Here's how the part is built. I have some questions about the finished solid (model axes, mm). Face numbers are marked on the shaded views. A direction names the side the tool comes from. Coordinates: 2 decimals unless noted, no trailing zeros. Order: outer loops, then holes, each group sorted by start corner. A loop starts at its lowest first (then second) coordinate and runs counter-clockwise, first axis right, second up. Notation, with made-up numbers: (34.5, -20.75) - (70.5, -20.75) arc R14 ccw to (70.5, -11.75) - close; hole circle Ø2 at (53.25, 82). An arc over 180 degrees is marked (long way). Use CSV: the item, a comma, the result in double quotes. Start each with the question number.
from build123d import *

# Parameters (mm, degrees)
F0_W      = 39.88
F0_H      = 19.82
F1_DEPTH  = 26.67
F2_W      = 6.48
F2_H      = 19.82
F2_W_2    = 39.88
F3_DEPTH  = 2
F4_W      = 39.88
F4_H      = 19.82
F5_DEPTH  = 7.35
F6_R      = 6
F7_DEPTH  = 1.8
F8_R      = 3
F8_R_2    = 1.3258580477
F9_DEPTH  = 4.05
F10_R     = 2.19
F11_DEPTH = 25
F12_R     = 2


with BuildPart() as f1:
    # F0 (on Top) → F1 (new body)
    with BuildSketch(Plane.XY):
        with Locations((19.94, 9.91)):
            Rectangle(F0_W, F0_H)
    extrude(amount=F1_DEPTH)

    # F2 (on face) → F3 (join)
    with BuildSketch(Plane.XY.offset(26.67)):
        with Locations((-3.24, 9.91)):
            Rectangle(F2_W, F2_H)
        with Locations((19.94, 9.91)):
            Rectangle(F2_W_2, F2_H)
        with Locations((43.12, 9.91)):
            Rectangle(F2_W, F2_H)
    extrude(amount=F3_DEPTH)

    # F4 (on face) → F5 (join)
    with BuildSketch(Plane.XY.offset(28.67)):
        with Locations((19.94, 9.91)):
            Rectangle(F4_W, F4_H)
    extrude(amount=F5_DEPTH)

    # F6 (on face) → F7 (join)
    with BuildSketch(Plane.XY.offset(36.02)):
        with Locations((9.66, 9.91)):
            Circle(F6_R)
    extrude(amount=F7_DEPTH)

    # F8 (on face) → F9 (join)
    with BuildSketch(Plane.XY.offset(37.82)):
        with Locations((9.66, 9.91)):
            Circle(F8_R)
        with Locations((9.66, 9.91)):
            Circle(F8_R_2, mode=Mode.SUBTRACT)
    extrude(amount=F9_DEPTH)

    # F10 (on face) → F11 (cut)
    with BuildSketch(Plane.XY.offset(28.67)):
        with Locations((-3.81, 4.825)):
            Circle(F10_R)
        with Locations((-3.81, 14.995)):
            Circle(F10_R)
        with Locations((43.69, 4.825)):
            Circle(F10_R)
        with Locations((43.69, 14.995)):
            Circle(F10_R)
    extrude(amount=-F11_DEPTH, mode=Mode.SUBTRACT)

    # F12
    f12_edges = [f1.edges().sort_by_distance(p)[0] for p in [
        (-6.48, 19.82, 27.67),
        (46.36, 19.82, 27.67),
        (46.36, 0, 27.67),
        (-6.48, 0, 27.67),
    ]]
    fillet(f12_edges, radius=F12_R)


solid = f1.part
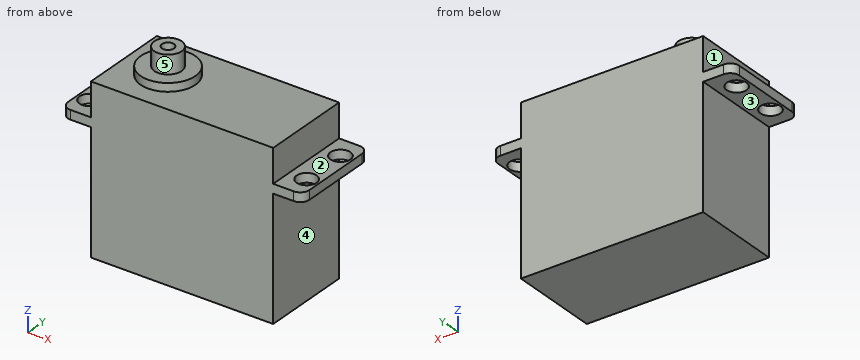
Item 1: For pin 1 Ø5 at (x, y) = (43.69, 14.995) entering from +Z; pin 2 Ø2 at (y, z) = (14, 33) entering from -X; pin 3 Ø10 at (x, y) = (18.5, 12) entering from +Z; pin 4 Ø2.5 at (x, y) = (-3.81, 4.825) entering from -Z, each with a flat end and sliding along its axis, tell me the tip position at first contact or that it passes through.
Item 2: Please list where these lines run through material, in increasing order: line 1 along Y through (x, z) = (43.69, 27.8) (3 decimals); line 2 along Y through (x, z) = (-3, 27); line 3 along X through (y, z) = (2.75, 9). Write a range as from..to.
Item 3: Suppose I cut it at D-D on x = 9.66. Write out the boundary of the cut face in (y, z), then the cut area to 3 significant figures.
Item 4: Suppose I cut it at A-A on x = -3.81. Write out the boundary of the cut face in (y, z) (3 decimals).
Item 5: Suppose I cut it at C-C on z = 28. Write out the boundary of the cut face in (x, y) (3 decimals).
Item 6: Suppose I cut it at B-B on y = 9.91. Write out the boundary of the cut face in (x, z).
Item 7: For the marked faces 1, 2, 3, 4 and 5, which set-ups out of +Z, -Z, +X, -X, +Y, -Y let a thin tool reach every point of the face, with its end or its side?
Here are the results:
1,pin 1,"z = 28.67"
1,pin 2,"x = 0"
1,pin 3,"z = 37.82"
1,pin 4,"through"
2,line 1,"0..2.635, 7.015..12.805, 17.185..19.82"
2,line 2,"0..2.79, 6.86..12.96, 17.03..19.82"
2,line 3,"0..39.88"
3,outline,"(0, 0) - (19.82, 0) - (19.82, 36.02) - (15.91, 36.02) - (15.91, 37.82) - (12.91, 37.82) - (12.91, 41.87) - (11.24, 41.87) - (11.24, 37.82) - (8.58, 37.82) - (8.58, 41.87) - (6.91, 41.87) - (6.91, 37.82) - (3.91, 37.82) - (3.91, 36.02) - (0, 36.02) - close"
3,area,"749 mm^2"
4,outline,"(0, 26.67) - (2.635, 26.67) - (2.635, 28.67) - (0, 28.67) - close; (7.015, 26.67) - (12.805, 26.67) - (12.805, 28.67) - (7.015, 28.67) - close; (17.185, 26.67) - (19.82, 26.67) - (19.82, 28.67) - (17.185, 28.67) - close"
5,outline,"(-6.48, 2) arc R2 ccw to (-4.48, 0) - (44.36, 0) arc R2 ccw to (46.36, 2) - (46.36, 17.82) arc R2 ccw to (44.36, 19.82) - (-4.48, 19.82) arc R2 ccw to (-6.48, 17.82) - close; hole circle Ø4.38 at (-3.81, 4.825); hole circle Ø4.38 at (-3.81, 14.995); hole circle Ø4.38 at (43.69, 4.825); hole circle Ø4.38 at (43.69, 14.995)"
6,outline,"(-6.48, 26.67) - (0, 26.67) - (0, 0) - (39.88, 0) - (39.88, 26.67) - (46.36, 26.67) - (46.36, 28.67) - (39.88, 28.67) - (39.88, 36.02) - (15.66, 36.02) - (15.66, 37.82) - (12.66, 37.82) - (12.66, 41.87) - (10.99, 41.87) - (10.99, 37.82) - (8.33, 37.82) - (8.33, 41.87) - (6.66, 41.87) - (6.66, 37.82) - (3.66, 37.82) - (3.66, 36.02) - (0, 36.02) - (0, 28.67) - (-6.48, 28.67) - close"
7,face 1,"+Z, -X, +Y, -Y"
7,face 2,"+Z, +X, +Y, -Y"
7,face 3,"-Z, -X, +Y, -Y"
7,face 4,"-Z, +X, +Y, -Y"
7,face 5,"+Z"
